Part model, mm, in its own coordinate system. Round coordinates to 2 decimals unless told otherwise and drop trailing zeros. Write each loop counter-clockwise with the first axis right and the second up, starting at its lowest first coordinate (ties: lowest second). Pieces come first, ordered by that corner, then holes. Notation, with made-up numbers: M 12,39.25 L 55,39.25 A28 cw 55,57.25 Z; hole C 75,-27.75 d1. An arc over 180 degrees is marked long. Use one line per item in the form item = value. Start each with the question number.
Item 1: Probe L1, parallel to Y at x = 0, z = 26; L2, parallel to Y at x = 2.5, z = 23; L3, parallel to Y at x = -0.5, z = 15. List the from-to ranges inside material, lowest first.
Item 2: Mould opens along X. For faces 1 (the face through (-2.586, 1.537, 34.51)), 2 (the face through (-1.89, -0.6, 76.45)), 3 (the face through (1, 1, 0)), 4 (the face through (-0.8, -0.6, 39.8)) say: +X half, -X half, draft (parallel to the pull), parting line (faces both ways), or undercut.
Item 3: Cut at A-A, the plane z = 31. Give the cut face in (x, y), then the cut area to 3 significant figures.
Item 4: Flat gauge pin, fed straight in: pin 1 Ø2 at (y, z) = (1, 33) entering from +X. Where does the tip first touch, or does it go through?
from build123d import *

# Parameters (mm, degrees)
F1_DEPTH = 70
F3_R     = 9.108661
F5_DEPTH = 85.001
F6_R     = 1.000895
F7_DEPTH = 85.001


with BuildPart() as f1:
    # F0 (on Top) → F1 (new body)
    with BuildSketch(Plane.XY):
        Polygon((-1.717262, 3.016132), (-3.47889, 0.016132), (-1.761628, -3.009482), (1.717262, -3.035097), (3.47889, -0.035097), (1.761628, 2.990518), align=None)
    extrude(amount=F1_DEPTH)

    # F2 (on Front) → F4 (revolve)
    with BuildSketch(Plane.XZ):
        Polygon((-3.47889, 70), (0, 70), (0, 85), align=None)
    revolve(axis=Axis((0, 0, 77.5), (0, 0, 1)))

    # F3 (on Top) → F5 (cut, through all)
    with BuildSketch(Plane.XY):
        with Locations((-4e-05, -0.009522)):
            Circle(F3_R)
        Polygon((-1.772364, -3.027722), (-3.50004, 0.016256), (-1.727715, 3.034456), (1.772285, 3.008678), (3.49996, -0.0353), (1.727636, -3.0535), align=None, mode=Mode.SUBTRACT)
    extrude(amount=F5_DEPTH, mode=Mode.SUBTRACT)

    # F6 (on Top) → F7 (cut, through all)
    with BuildSketch(Plane.XY):
        Circle(F6_R)
    extrude(amount=F7_DEPTH, mode=Mode.SUBTRACT)


solid = f1.part
Model answer:
q1.L1 = -3.02 to -1, 1 to 3
q1.L2 = -1.7 to 1.69
q1.L3 = -3.02 to -0.87, 0.87 to 3.01
q2.face_1 = -X half
q2.face_2 = parting line
q2.face_3 = draft
q2.face_4 = undercut
q3.outline = M -3.48,0.02 L -1.76,-3.01 L 1.72,-3.04 L 3.48,-0.04 L 1.76,2.99 L -1.72,3.02 Z; hole C 0,0 d2
q3.area = 28.3 mm²
q4.pin_1 = 3.46
